Source: CAD feature listing. Evaluate the final solid. Frame: model axes, mm. Face numbers are marked on the shaded views. Round coordinates to 2 decimals unless told otherwise and drop trailing zeros. Return JSON: item names as keys, results as strings. Group by question number.
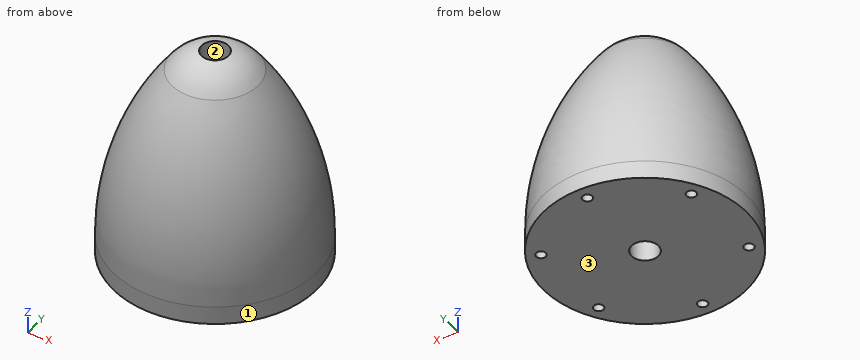
```python
from build123d import *

# Parameters (mm, degrees)
F0_R     = 35.9791
F1_DEPTH = 76.2
F4_R     = 4.7625
F5_DEPTH = 156
F6_R     = 1.7272
F7_DEPTH = 12.7


# Not quite as in the source:
# - an extrude ends at something that could not be found from the text; its depth is read off the source's solid


with BuildPart() as f1:
    # F0 (on Top) → F1 (new body)
    with BuildSketch(Plane.XY):
        Circle(F0_R)
    extrude(amount=F1_DEPTH)

    # F2 (on Front) → F3 (revolve, cut)
    with BuildSketch(Plane.XZ):
        with BuildLine():
            ThreePointArc((0, 76.2), (8.5206969151, 74.1881989682), (15.2417143714, 68.5777138143))
            ThreePointArc((15.2417143714, 68.5777138143), (30.6582935654, 39.1460650432), (35.9791, 6.35))
            Line((35.9791, 6.35), (71.9582, 6.35))
            Line((71.9582, 6.35), (71.9582, 112.1791))
            Line((71.9582, 112.1791), (0, 112.1791))
            Line((0, 112.1791), (0, 76.2))
        make_face()
    revolve(axis=Axis((0, 0, 76.2), (0, 0, 1)), mode=Mode.SUBTRACT)

    # F4 (on face) → F5 (cut, through all)
    with BuildSketch(Plane(origin=(0, 0, 0), x_dir=(1, 0, 0), z_dir=(0, 0, -1))):
        Circle(F4_R)
    extrude(amount=-F5_DEPTH, mode=Mode.SUBTRACT)

    # F6 (on face) → F7 (cut)
    with BuildSketch(Plane(origin=(0, 0, 0), x_dir=(1, 0, 0), z_dir=(0, 0, -1))):
        with Locations((-27.0343686198, -15.6083)):
            Circle(F6_R)
        with Locations((-27.0343686198, 15.6083)):
            Circle(F6_R)
        with Locations((0, 31.2166)):
            Circle(F6_R)
        with Locations((27.0343686198, 15.6083)):
            Circle(F6_R)
        with Locations((27.0343686198, -15.6083)):
            Circle(F6_R)
        with Locations((0, -31.2166)):
            Circle(F6_R)
    extrude(amount=-F7_DEPTH, mode=Mode.SUBTRACT)


solid = f1.part
```
(1) Pin query (flat end, axial travel): pin 1 (4 mm diameter, centred on x = 27.5, y = 15.5, fed in from -Z); pin 2 (3 mm diameter, centred on x = 0, y = 31.22, fed in from -Z); pin 3 (10 mm diameter, centred on y = 8.5, z = 62.5, fed in from -X); pin 4 (5 mm diameter, centred on x = 23.5, z = 42.5, fed in from +Y). Return the tip coordinate at first contact, or that it passes through.
(2) Mould query, pull axis Y, two halves, no side actions, for the marked faces 1, 2 and 3. Classes: released by +Y, released by -Y, zero draft, split by the parting line, or undercut.
(3) Ray query, line 1 (Y direction, x = 0, z = 3); line 2 (Y direction, x = 25.5, z = 7); line 3 (Y direction, x = -2, z = 28). Return the intervals inside material, ascending.
Answers follow:
{
 "1": {"pin 1": "z = 0", "pin 2": "z = 12.7", "pin 3": "x = -21.29", "pin 4": "y = 21"},
 "2": {"face 1": "split by the parting line", "face 2": "undercut", "face 3": "zero draft"},
 "3": {"line 1": "-35.98 to -32.94, -29.49 to -4.76, 4.76 to 29.49, 32.94 to 35.98", "line 2": "-25.38 to -16.4, -14.82 to 14.82, 16.4 to 25.38", "line 3": "-33.64 to -4.32, 4.32 to 33.64"}
}
